from build123d import *

# Parameters (mm, degrees)
SKETCH_1_R           = 25
SKETCH_1_R_2         = 20
EXTRUDE_1_DEPTH      = 1.6
EXTRUDE_START        = -6
SKETCH_4_R           = 20
SKETCH_4_R_2         = 25
EXTRUDE_2_DEPTH      = 6
SKETCH_5_OUTSIDE_W   = 222.406
SKETCH_5_OUTSIDE_H   = 191.906
SKETCH_5_OUTSIDE_W_2 = 148.6
SKETCH_5_OUTSIDE_H_2 = 200
CUT_EXTRUDE_1_DEPTH  = 10
SKETCH_6_R           = 5
CUT_EXTRUDE_2_DEPTH  = 10
SKETCH_8_W           = 10
SKETCH_8_H           = 25
CUT_EXTRUDE_4_DEPTH  = 10
SKETCH_9_R           = 1.5
CUT_EXTRUDE_5_DEPTH  = 116.180128425


with BuildPart() as part:
    # 草图1 → 凸台-拉伸1 (new body)
    with BuildSketch(Plane.XY):
        with BuildLine():
            Line((-66.387122245, 57), (66.387122245, 57))
            ThreePointArc((66.387122245, 57), (0, -87.5), (-66.387122245, 57))
        make_face()
        Circle(SKETCH_1_R, mode=Mode.SUBTRACT)
        with Locations((54.772, 35)):
            Circle(SKETCH_1_R_2, mode=Mode.SUBTRACT)
        with Locations(Location((-54.772, 35, 0), (0, 0, 180))):
            Circle(SKETCH_1_R_2, mode=Mode.SUBTRACT)
        with Locations((35, -54.772)):
            Circle(SKETCH_1_R_2, mode=Mode.SUBTRACT)
        with Locations((-35, -54.772)):
            Circle(SKETCH_1_R_2, mode=Mode.SUBTRACT)
    extrude(amount=EXTRUDE_1_DEPTH)

    # 草图4 → 凸台-拉伸2 (add)
    with BuildSketch(Plane.XY.offset(1.6).offset(EXTRUDE_START)):
        with Locations((-54.772, 35)):
            Circle(SKETCH_4_R)
        Circle(SKETCH_4_R_2)
        with Locations((54.772, 35)):
            Circle(SKETCH_4_R)
        with Locations((-35, -54.772)):
            Circle(SKETCH_4_R)
        with Locations((35, -54.772)):
            Circle(SKETCH_4_R)
    extrude(amount=EXTRUDE_2_DEPTH)

    # 草图5 outside → 切除-拉伸1 (cut)
    with BuildSketch(Plane(origin=(0, 0, 0), x_dir=(-1, 0, 0), z_dir=(0, 0, -1))):
        with Locations((0, -15.25)):
            Rectangle(SKETCH_5_OUTSIDE_W, SKETCH_5_OUTSIDE_H)
        Rectangle(SKETCH_5_OUTSIDE_W_2, SKETCH_5_OUTSIDE_H_2, mode=Mode.SUBTRACT)
    extrude(amount=-CUT_EXTRUDE_1_DEPTH, mode=Mode.SUBTRACT)

    # 草图6 → 切除-拉伸2 (cut)
    with BuildSketch(Plane(origin=(0, 0, 0), x_dir=(-1, 0, 0), z_dir=(0, 0, -1))):
        with Locations((-77, -27)):
            Circle(SKETCH_6_R)
        with Locations((-77, 26)):
            Circle(SKETCH_6_R)
        with Locations((77, 26)):
            Circle(SKETCH_6_R)
        with Locations((77, -27)):
            Circle(SKETCH_6_R)
    extrude(amount=-CUT_EXTRUDE_2_DEPTH, mode=Mode.SUBTRACT)

    # 草图8 → 切除-拉伸4 (cut)
    with BuildSketch(Plane.XY.offset(1.6)):
        with Locations((-42.3, -10)):
            Rectangle(SKETCH_8_W, SKETCH_8_H)
    extrude(amount=-CUT_EXTRUDE_4_DEPTH, mode=Mode.SUBTRACT)

    # 草图9 → 切除-拉伸5 (cut, through all)
    with BuildSketch(Plane(origin=(0, 0, 0), x_dir=(-1, 0, 0), z_dir=(0, 0, -1))):
        with Locations((-71, 20)):
            Circle(SKETCH_9_R)
        with Locations((-71, -22)):
            Circle(SKETCH_9_R)
        with Locations((71, 20)):
            Circle(SKETCH_9_R)
        with Locations((71, -22)):
            Circle(SKETCH_9_R)
    extrude(amount=-CUT_EXTRUDE_5_DEPTH, mode=Mode.SUBTRACT)


solid = part.part
Can you work these out from the model? Positions are in its coordinate system, mm. A direction names the side the tool comes from. Coordinates: 2 decimals unless noted, no trailing zeros. Write each loop counter-clockwise with the first axis right and the second up, starting at its lowest first coordinate (ties: lowest second). Pieces come first, ordered by that corner, then holes. Notation, with made-up numbers: (76.5, 12) -> (87.5, 12) arc R24 ccw to (87.5, 31) -> close; hole circle Ø3 at (-6.75, 9.25). An arc over 180 degrees is marked (long way). Answer as CSV lines item,"result".
1) On a 3-axis mill with a long thin cutter (end or side, diameter ignored), from which of +Z, -Z, +X, -X, +Y, -Y can I reach the whole of each face in a straight line? I mean faces 1 (the cylindrical face through (-35.696, 41.007, -2.231)), 2 (the flat face through (54, 35, -4.4)). Say none if no direction works.
Check result:
face 1,"-Z"
face 2,"-Z, +X, -X, +Y, -Y"
2) If we section it at A-A on y = 0: Please give me the cut outline in (x, z), then the cut area to 3 significant figures.
Check result:
outline,"(-74.3, 0) -> (-47.3, 0) -> (-47.3, 1.6) -> (-74.3, 1.6) -> close; (-37.3, 0) -> (-25, 0) -> (-25, -4.4) -> (25, -4.4) -> (25, 0) -> (74.3, 0) -> (74.3, 1.6) -> (-37.3, 1.6) -> close"
area,"442 mm²"
3) Will these pins go through, and if not, where does the flat tip stop? P1, Ø1.5, axis at x = -21, z = -3.5, coming from the +Y side; P2, Ø2.5, axis at x = -71, y = -22, coming from the -Z side; P3, Ø1.8, axis at x = -42.5, z = 1, coming from the -Y side; P4, Ø2.5, axis at x = 73.5, y = 26.5, coming from the +Z side.
Check result:
P1,"y = 14.66"
P2,"through"
P3,"y = -76.98"
P4,"z = 0"
4) If we section it at C-C on y = -18: Please give me the cut outline in (x, z), then the cut area to 3 significant figures.
Check result:
outline,"(-74.3, 0) -> (-47.3, 0) -> (-47.3, 1.6) -> (-74.3, 1.6) -> close; (-37.3, 0) -> (-17.35, 0) -> (-17.35, -4.4) -> (17.35, -4.4) -> (17.35, 0) -> (74.3, 0) -> (74.3, 1.6) -> (-37.3, 1.6) -> close"
area,"374 mm²"
5) If we section it at B-B on x = 29.5: Please give me the cut outline in (y, z).
Check result:
outline,"(-82.38, 0) -> (-74, 0) -> (-74, -4.4) -> (-35.54, -4.4) -> (-35.54, 0) -> (57, 0) -> (57, 1.6) -> (-82.38, 1.6) -> close"
6) If we section it at D-D on y = -43.5: Please give me the cut outline in (x, z).
Check result:
outline,"(-74.3, 0) -> (-51.52, 0) -> (-51.52, -4.4) -> (-18.48, -4.4) -> (-18.48, 0) -> (18.48, 0) -> (18.48, -4.4) -> (51.52, -4.4) -> (51.52, 0) -> (74.3, 0) -> (74.3, 1.6) -> (-74.3, 1.6) -> close"
7) If I drill on line 1 (X direction, y = 35, z = -3.4); line 2 (Y direction, x = 71, z = 0.4); line 3 (Z direction, x = 41, y = -30), over which ranges is the centre line in solid material (lowest first)? Write a range as from..to.
Check result:
line 1,"-74.77..-34.77, 34.77..74.77"
line 2,"-51.14..-23.5, -20.5..18.5, 21.5..51.14"
line 3,"0..1.6"
